Autodesk Inventor part; units mm, degrees
ref_plane "to_at504_knurled_face_nut_XY" through (0, 2.5146, 0) normal (0, -1, 0) x (1, 0, 0)
ref_plane "to_at504_knurled_face_nut_YZ" through (0, 2.5146, 0) normal (1, 0, 0) x (0, 0, 1)
ref_plane "to_at504_knurled_face_nut_ZX" through (0, 2.5146, 0) normal (0, 0, 1) x (0, -1, 0)
sketch "Sketch_2" plane through (0, 0, 0) normal (1, 0, 0) x (0, 1, 0)
  line L0 (0, 0) -> (8.9916, 0)
  line L1 (8.4836, 0) -> (8.4836, -4.2037)
  line L2 (8.4836, -4.2037) -> (8.9916, -4.2037)
  line L3 (8.9916, -4.2037) -> (8.9916, -4.9265)
  line L4 (8.9916, -4.9265) -> (7.9181, -6)
  line L5 (7.9181, -6) -> (0, -6)
  line L6 (0, -6) -> (0, 0)
  line L7 (0, 0) -> (8.4836, 0)
revolve "Revolution1" add sketch "Sketch_2" angle 360 about axis through (0, 0, 0) along (0, -1, 0)
sketch "Sketch_3" plane through (0, 0, 0) normal (1, 0, 0) x (0, 1, 0)
  line L0 (-5.0292, 0) -> (0, 0)
  line L1 (0, 0) -> (0, -6)
  line L2 (0, -6) -> (-4.5212, -6)
  arc A0 (-5.0292, -5.492) -> (-4.5212, -6) centre (-4.5212, -5.492) ccw
  line L3 (-5.0292, -5.492) -> (-5.0292, 0)
  line L4 (-5.0292, 0) -> (0, 0)
revolve "Revolution2" add sketch "Sketch_3" angle 360 about axis through (0, -5.0292, 0) along (0, -1, 0)
sketch "Sketch_7" plane through (0, 0, 0) normal (1, 0, 0) x (0, 1, 0)
  line L0 (-5.2832, 0) -> (-0.254, 0)
  line L1 (-0.254, 0) -> (-0.254, -5.7404)
  line L2 (-0.254, -5.7404) -> (-4.2672, -5.7404)
  arc A0 (-4.7752, -5.2324) -> (-4.2672, -5.7404) centre (-4.2672, -5.2324) ccw
  line L3 (-4.7752, -5.2324) -> (-4.7752, -4.9784)
  line L4 (-4.7752, -4.9784) -> (-5.2832, -4.9784)
  line L5 (-5.2832, -4.9784) -> (-5.2832, 0)
  line L6 (-5.2832, 0) -> (-0.254, 0)
sketch "Sketch_9" plane through (0, -5.0292, 0) normal (0, 1, 0) x (1, 0, 0)
  line L0 (-11.646, -2.8576) -> (-11.5146, -3.3483)
  line L1 (-11.5146, -3.3483) -> (11.646, 2.8576)
  line L2 (11.646, 2.8576) -> (11.5146, 3.3483)
  line L3 (11.5146, 3.3483) -> (-11.646, -2.8576)
extrude "Extrusion1" cut sketch "Sketch_9" along normal blind 0.762
revolve "Revolution3" cut sketch "Sketch_7" angle 360 about axis through (0, -5.2832, 0) along (0, -1, 0)
ref_plane "to_at504_knurled_face_nut_XY" through (0, 2.5146, 0) normal (0, -1, 0) x (1, 0, 0)
ref_plane "to_at504_knurled_face_nut_YZ" through (0, 2.5146, 0) normal (1, 0, 0) x (0, 0, 1)
ref_plane "to_at504_knurled_face_nut_ZX" through (0, 2.5146, 0) normal (0, 0, 1) x (0, -1, 0)
ref_plane "to_at508_lockwasher_XY" through (0, 2.0066, 0) normal (0, 1, 0) x (1, 0, 0)
ref_plane "to_at508_lockwasher_YZ" through (0, 2.0066, 0) normal (1, 0, 0) x (0, 0, -1)
ref_plane "to_at508_lockwasher_ZX" through (0, 2.0066, 0) normal (0, 0, -1) x (0, 1, 0)
ref_plane "to_dummy_XY" through (0, 0, 0) normal (0, -1, 0) x (1, 0, 0)
ref_plane "to_dummy_YZ" through (0, 0, 0) normal (1, 0, 0) x (0, 0, 1)
ref_plane "to_dummy_ZX" through (0, 0, 0) normal (0, 0, 1) x (0, -1, 0)
ref_plane "to_hex_nut_XY" through (0, 0, 0) normal (0, 1, 0) x (1, 0, 0)
ref_plane "to_hex_nut_YZ" through (0, 0, 0) normal (1, 0, 0) x (0, 0, -1)
ref_plane "to_hex_nut_ZX" through (0, 0, 0) normal (0, 0, -1) x (0, 1, 0)
ref_plane "to_plunger_XY" through (0, 8.9916, 0) normal (0, -1, 0) x (1, 0, 0)
ref_plane "to_plunger_YZ" through (0, 8.9916, 0) normal (1, 0, 0) x (0, 0, 1)
ref_plane "to_plunger_ZX" through (0, 8.9916, 0) normal (0, 0, 1) x (0, -1, 0)
ref_plane "to_trmnl_hold_XY" through (0, -5.0292, 0) normal (0, 1, 0) x (1, 0, 0)
ref_plane "to_trmnl_hold_YZ" through (0, -5.0292, 0) normal (1, 0, 0) x (0, 0, -1)
ref_plane "to_trmnl_hold_ZX" through (0, -5.0292, 0) normal (0, 0, -1) x (0, 1, 0)
properties part number "SB4011NOM-body"
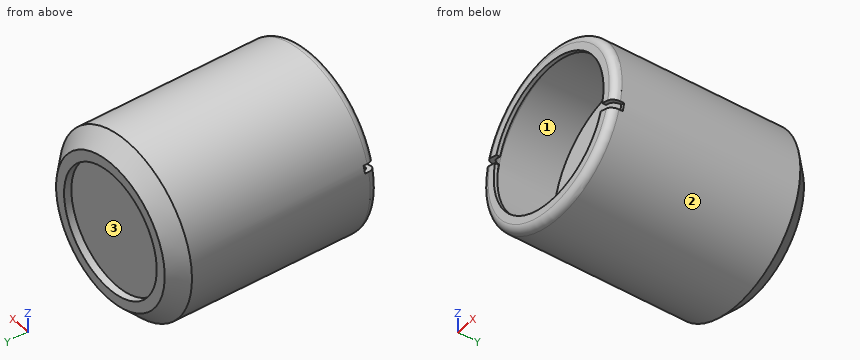
Geometry: final body of the model. Coordinates: model frame, mm. Face numbers are marked on the shaded views. Round coordinates to 2 decimals unless told otherwise and drop trailing zeros. Loops run counter-clockwise (first coordinate to the right, second up) from the corner with the lowest first, then second, coordinate; pieces in that order, holes last.
Q1. Material intervals for L1, parallel to X at y = -3.1, z = 0; L2, parallel to Y at x = -0.5, z = -4.5, sorted ascending.
Q2. Section B-B on z = 0. Return loops of the section in (x, y), plus the area to 3 significant figures.
Q3. Section A-A on x = 0. Return loops of the section in (y, z), plus the area to 3 significant figures.
Q4. Section C-C on y = -1.75. Return loops of the section in (x, z), plus the area to 3 significant figures.
Q5. Pin query (flat end, axial travel): P1, Ø3, axis at x = 1, y = 5.5, coming from the +Z side; P2, Ø1.9, axis at x = 0, z = -1.5, coming from the +Y side; P3, Ø1.5, axis at y = 7.5, z = -4.5, coming from the -X side; P4, Ø4, axis at x = -3, y = -1.5, coming from the +Z side. Return the tip coordinate at first contact, or that it passes through.
Q6. Pull-direction query (X, two-part tool) for the marked faces 1, 2 and 3; classes: released by +X, released by -X, zero draft, split by the parting line, or undercut.
Q7. Section D-D on y = 1.5. Return loops of the section in (x, z).
Evaluation:
1. L1: x = -6 to -5.74, 5.74 to 6
1. L2: y = -0.25 to 8.99
2. outline: (-6, -4.52) arc R0.51 ccw to (-5.49, -5.03) - (-4.98, -5.03) - (-4.98, -4.78) - (-5.23, -4.78) arc R0.51 cw to (-5.74, -4.27) - (-5.74, -0.25) - (5.74, -0.25) - (5.74, -4.27) arc R0.51 cw to (5.23, -4.78) - (4.98, -4.78) - (4.98, -5.03) - (5.49, -5.03) arc R0.51 ccw to (6, -4.52) - (6, 7.92) - (4.93, 8.99) - (4.2, 8.99) - (4.2, 8.48) - (-4.2, 8.48) - (-4.2, 8.99) - (-4.93, 8.99) - (-6, 7.92) - close
2. area: 108 mm2
3. outline: (-5.03, -5.49) arc R0.51 ccw to (-4.52, -6) - (7.92, -6) - (8.99, -4.93) - (8.99, -4.2) - (8.48, -4.2) - (8.48, 4.2) - (8.99, 4.2) - (8.99, 4.93) - (7.92, 6) - (-4.52, 6) arc R0.51 ccw to (-5.03, 5.49) - (-5.03, 4.98) - (-4.78, 4.98) - (-4.78, 5.23) arc R0.51 cw to (-4.27, 5.74) - (-0.25, 5.74) - (-0.25, -5.74) - (-4.27, -5.74) arc R0.51 cw to (-4.78, -5.23) - (-4.78, -4.98) - (-5.03, -4.98) - close
3. area: 108 mm2
4. outline: circle Ø12 at (0, 0); hole circle Ø11.48 at (0, 0)
4. area: 9.57 mm2
5. P1: stops at z = 6
5. P2: stops at y = 8.48
5. P3: stops at x = -4.68
5. P4: stops at z = 5.92
6. face 1: undercut
6. face 2: split by the parting line
6. face 3: undercut
7. outline: circle Ø12 at (0, 0)
